from build123d import *

# Parameters (mm, degrees)
SKETCH1_R           = 1.25
SKETCH1_R_2         = 1.250329794
SKETCH1_R_3         = 1.7
BOSS_EXTRUDE1_DEPTH = 5
SKETCH2_R           = 1.7
SKETCH2_W           = 44.709414805
SKETCH2_H           = 5.189
BOSS_EXTRUDE2_DEPTH = 5


with BuildPart() as part:
    # Sketch1 → Boss-Extrude1 (new body)
    with BuildSketch(Plane.XY):
        Polygon((85.253810187, 98.97317398), (129.963224992, 98.97317398), (129.963224992, 93.786173942), (132.040225419, 93.78317398), (132.040225419, 53.78317398), (129.963224992, 53.78317398), (129.963224992, 48.59417398), (85.253810187, 48.59417398), align=None)
        with Locations((129.540225419, 91.28317398)):
            Circle(SKETCH1_R, mode=Mode.SUBTRACT)
        with Locations((129.540225419, 56.254458242)):
            Circle(SKETCH1_R_2, mode=Mode.SUBTRACT)
        with Locations((121.835225419, 51.56417398)):
            Circle(SKETCH1_R_3, mode=Mode.SUBTRACT)
        with Locations((121.835225419, 96.00317398)):
            Circle(SKETCH1_R_3, mode=Mode.SUBTRACT)
    extrude(amount=BOSS_EXTRUDE1_DEPTH)

    # Sketch2 → Boss-Extrude2 (add)
    # profile 1 of 2: a face of its own
    with BuildSketch(Plane.XY.offset(5)):
        Polygon((129.963224992, 93.786173942), (85.253810187, 93.78317398), (85.253810187, 98.97317398), (129.963224992, 98.97317398), align=None)
        with Locations((121.835225419, 96.00317398)):
            Circle(SKETCH2_R, mode=Mode.SUBTRACT)
    # profile 2 of 2: a face of its own
    with BuildSketch(Plane.XY.offset(5)):
        with Locations((107.60851759, 51.18867398)):
            Rectangle(SKETCH2_W, SKETCH2_H)
        with Locations((121.835225419, 51.56417398)):
            Circle(SKETCH2_R, mode=Mode.SUBTRACT)
    extrude(amount=BOSS_EXTRUDE2_DEPTH)


solid = part.part
Work out the finished part from the listing and answer in its coordinate system (mm). A direction names the side the tool comes from. Round coordinates to 2 decimals unless told otherwise and drop trailing zeros. Write each loop counter-clockwise with the first axis right and the second up, starting at its lowest first coordinate (ties: lowest second). Pieces come first, ordered by that corner, then holes.
1) Given pin 1 Ø10 at (x, y) = (109.5, 81) entering from +Z; pin 2 Ø2.5 at (x, y) = (121.84, 96) entering from -Z; pin 3 Ø1.6 at (y, z) = (51, 7.5) entering from +X; pin 4 Ø1 at (x, z) = (131, 2) entering from -Y, each flat-ended and moving along its own axis, determine where each tip first touches the part or whether it passes through.
2) A tool of negligible diameter and unlimited length cuts with its end or side. For faces 1 (the flat face through (131, 53.783, 2)), 2 (the flat face through (129.963, 96, 5)), 3 (the flat face through (109, 74, 5)), from which of +Z, -Z, +X, -X, +Y, -Y can it reach the whole face along a straight path? Write none if from no direction.
3) A cutting plane is placed at B-B (x = 94). Give the vertices of the cut face in (y, z), plus the area to 3 significant figures.
4) The mould has two halves that part along Y. Classify faces 4 (the flat face through (107, 98.973, 5)), 5 (the cylindrical face through (120.137, 51.639, 4.93)), 6 (the flat face through (108, 96, 10)): pulls with the +Y half, pulls with the -Y half, needs draft (parallel to the pull), parting line crosses it, or undercut.
5) A cutting plane is placed at C-C (y = 68). Give the vertices of the cut face in (x, z).
6) Straight lines are drawn through the part: line 1 (X direction, y = 96, z = 2); line 2 (Y direction, x = 112, z = 8.5); line 3 (Z direction, x = 125.5, y = 88.5). For each, find the intervals that lie inside material, in ascending order.
7) A cutting plane is placed at A-A (z = 8.5). Give the vertices of the cut face in (x, y).
8) A cutting plane is placed at D-D (z = 2.75). Give the vertices of the cut face in (x, y), plus the area to 3 significant figures.
Completed:
1. pin 1: stops at z = 5
1. pin 2: passes through
1. pin 3: stops at x = 129.96
1. pin 4: stops at y = 53.78
2. face 1: +Z, -Z, +X, -Y
2. face 2: +Z, -Z, +X, +Y
2. face 3: +Z, +X, -X
3. outline: (48.59, 0) - (98.97, 0) - (98.97, 10) - (93.78, 10) - (93.78, 5) - (53.78, 5) - (53.78, 10) - (48.59, 10) - close
3. area: 304 mm2
4. face 4: pulls with the +Y half
4. face 5: undercut
4. face 6: needs draft
5. outline: (85.25, 0) - (132.04, 0) - (132.04, 5) - (85.25, 5) - close
6. line 1: x = 85.25 to 120.14, 123.54 to 129.96
6. line 2: y = 48.59 to 53.78, 93.78 to 98.97
6. line 3: z = 0 to 5
7. outline: (85.25, 48.59) - (129.96, 48.59) - (129.96, 53.78) - (85.25, 53.78) - close; (85.25, 93.78) - (129.96, 93.79) - (129.96, 98.97) - (85.25, 98.97) - close; hole circle Ø3.4 at (121.84, 51.56); hole circle Ø3.4 at (121.84, 96)
8. outline: (85.25, 48.59) - (129.96, 48.59) - (129.96, 53.78) - (132.04, 53.78) - (132.04, 93.78) - (129.96, 93.79) - (129.96, 98.97) - (85.25, 98.97) - close; hole circle Ø3.4 at (121.84, 51.56); hole circle Ø3.4 at (121.84, 96); hole circle Ø2.5 at (129.54, 56.25); hole circle Ø2.5 at (129.54, 91.28)
8. area: 2,310 mm2
